from build123d import *

# Parameters (mm, degrees)
F0_W      = 116
F0_H      = 58
F1_DEPTH  = 80
F2_T      = -3
F4_DEPTH  = 47
F5_R      = 2
F6_DEPTH  = 3.001
F7_W      = 58
F7_H      = 4
F8_DEPTH  = 15
F9_R      = 10
F10_R     = 2
F11_DEPTH = 4.001
F12_W     = 48
F12_H     = 28.5
F13_DEPTH = 5
F14_R     = 1.875
F15_DEPTH = 5
F16_W     = 25
F16_H     = 5
F17_DEPTH = 5.001
F18_R     = 2.49999
F19_R     = 2.5
F20_SIZE  = 7


# Not quite as in the source:
# - a fillet or chamfer is up to 0.001 mm smaller than in the source, because OpenCascade refuses the exact size
# - a pattern or mirror of a feature is missing from the dataset's text; its kind, count and spacing are read off the source's solid


with BuildPart() as f1:
    # F0 (on Top) → F1 (new body)
    with BuildSketch(Plane.XY):
        Rectangle(F0_W, F0_H)
    extrude(amount=F1_DEPTH)

    # F2
    f2_openings = [f1.faces().sort_by_distance(p)[0] for p in [
        (0, 0, 80),
    ]]
    offset(amount=F2_T, openings=f2_openings)

    # F3 (on face) → F4 (join)
    with BuildSketch(Plane.XY.offset(3)):
        Polygon((-55, 26), (-55, 24), (53, 24), (53, -26), (55, -26), (55, 26), align=None)
    extrude(amount=F4_DEPTH)

    # F5 (on face) → F6 (cut, through all)
    with BuildSketch(Plane(origin=(55, 0, 0), x_dir=(0, -1, 0), z_dir=(-1, 0, 0))):
        with Locations((0, 69)):
            Circle(F5_R)
    extrude(amount=-F6_DEPTH, mode=Mode.SUBTRACT)

    # F7 (on face) → F8 (join)
    with BuildSketch(Plane.YZ.offset(58)):
        with Locations((0, 2)):
            Rectangle(F7_W, F7_H)
    f8 = extrude(amount=F8_DEPTH)

    # F8_copies: F8 across plane
    add(f8.mirror(Plane(origin=(0, 0, 0), x_dir=(0, 0, -1), z_dir=(-1, 0, 0))))

    # F9
    f9_edges = [f1.edges().sort_by_distance(p)[0] for p in [
        (73, 29, 2),
        (73, -29, 2),
        (-73, -29, 2),
        (-73, 29, 2),
    ]]
    fillet(f9_edges, radius=F9_R)

    # F10 (on face) → F11 (cut, through all)
    with BuildSketch(Plane.XY.offset(4)):
        with Locations((64.8827031255, 16)):
            Circle(F10_R)
        with Locations((64.8827031255, -16)):
            Circle(F10_R)
    f11 = extrude(amount=-F11_DEPTH, mode=Mode.SUBTRACT)

    # F11_copies: F11 across plane
    add(f11.mirror(Plane(origin=(0, 0, 0), x_dir=(0, 0, -1), z_dir=(-1, 0, 0))), mode=Mode.SUBTRACT)

    # F12 (on face) → F13 (cut)
    with BuildSketch(Plane.XZ.offset(29)):
        with Locations((-27, 26.25)):
            Rectangle(F12_W, F12_H)
    extrude(amount=-F13_DEPTH, mode=Mode.SUBTRACT)

    # F14 (on face) → F15 (cut)
    with BuildSketch(Plane.XZ.offset(29)):
        with Locations((-27, 47.1)):
            Circle(F14_R)
        with Locations((-27, 5.4)):
            Circle(F14_R)
    extrude(amount=-F15_DEPTH, mode=Mode.SUBTRACT)

    # F16 (on face) → F17 (cut, through all)
    with BuildSketch(Plane.XZ.offset(-24)):
        with Locations((20.5, 10.5)):
            Rectangle(F16_W, F16_H)
    extrude(amount=-F17_DEPTH, mode=Mode.SUBTRACT)

    # F18 (radius 2.5 in the source; OpenCascade refuses exactly that, so slightly less here)
    f18_edges = [f1.edges().sort_by_distance(p)[0] for p in [
        (33, 26.5, 13),
        (8, 26.5, 13),
        (33, 26.5, 8),
        (8, 26.5, 8),
    ]]
    fillet(f18_edges, radius=F18_R)

    # F19
    f19_edges = [f1.edges().sort_by_distance(p)[0] for p in [
        (-58, -29, 42),
        (58, -29, 42),
        (58, 29, 42),
        (-58, 29, 42),
    ]]
    fillet(f19_edges, radius=F19_R)

    # F20
    f20_edges = [f1.edges().sort_by_distance(p)[0] for p in [
        (-55, -1, 3),
        (53, -1, 3),
    ]]
    chamfer(f20_edges, length=F20_SIZE)


solid = f1.part
CAD build for the part. Positions are in the model's coordinates, mm. A direction names the side the tool comes from. Round coordinates to 2 decimals unless told otherwise and drop trailing zeros. Loops run counter-clockwise (first coordinate to the right, second up) from the corner with the lowest first, then second, coordinate; pieces in that order, holes last.
(1) Which spindle directions (+Z, -Z, +X, -X, +Y, -Y) get a long thin tool onto all of the face, cutting with end or side? Do faces 4 (the flat face through (20, 26, 13)), 5 (the cylindrical face through (56, 0, 71)), 6 (the flat face through (53, -1, 30)), 7 (the flat face through (-51, -28, 26)). Say none if no direction does.
(2) Cut at A-A (x = 26.5). Give the cut face in (y, z), plus the area to 3 significant figures.
(3) Cut at D-D (z = 23). Give the cut face in (x, y), plus the area to 3 significant figures.
(4) Cut at C-C (z = 73). Give the cut face in (x, y), plus the area to 3 significant figures.
(5) Two-plate mould, pull along Y, no slides. Class faces 1 (the flat face through (-1, 26, 65)), 2 (the cylindrical face through (-25.27, -27.52, 46.38)), 3 (the cylindrical face through (-69.99, -26.15, 2.03)): +Y half, -Y half, draft (parallel to the pull), parting line (faces both ways), or undercut.
(6) Cut at B-B (y = -16). Give the cut face in (x, z).
(7) Drop flat-ended pins along their axis: pin 1 (3.5 mm diameter, centred on x = -64.88, y = -16, fed in from -Z); pin 2 (4.5 mm diameter, centred on x = 64.88, y = 16, fed in from +Z); pin 3 (16 mm diameter, centred on y = 8, z = 47, fed in from -X); pin 4 (1.5 mm diameter, centred on y = -11.5, z = 68.5, fed in from +X). Give the stop position or say it passes through.
(8) Wall check: line 1 along X through (y, z) = (15, 47.5); line 2 along Y through (x, z) = (28, 38.5); line 3 along X through (y, z) = (-1.5, 59). Give the ranges that are in metal, low to high.
Findings below:
1. face 4: +Y
1. face 5: +X
1. face 6: +Z
1. face 7: -Y
2. outline: (-29, 0) - (29, 0) - (29, 8) - (24, 8) - (24, 3) - (-26, 3) - (-26, 80) - (-29, 80) - close; (24, 13) - (29, 13) - (29, 80) - (26, 80) - (26, 50) - (24, 50) - close
2. area: 705 mm2
3. outline: (-58, -26.5) arc R2.5 ccw to (-55.5, -29) - (-51, -29) - (-51, -26) - (-55, -26) - (-55, 24) - (53, 24) - (53, -26) - (-3, -26) - (-3, -29) - (55.5, -29) arc R2.5 ccw to (58, -26.5) - (58, 26.5) arc R2.5 ccw to (55.5, 29) - (-55.5, 29) arc R2.5 ccw to (-58, 26.5) - close
3. area: 1,180 mm2
4. outline: (-58, -26.5) arc R2.5 ccw to (-55.5, -29) - (55.5, -29) arc R2.5 ccw to (58, -26.5) - (58, 26.5) arc R2.5 ccw to (55.5, 29) - (-55.5, 29) arc R2.5 ccw to (-58, 26.5) - close; hole (-55, -26) - (55, -26) - (55, 26) - (-55, 26) - close
4. area: 1,000 mm2
5. face 1: undercut
5. face 2: draft
5. face 3: -Y half
6. outline: (-73, 0) - (-66.88, 0) - (-66.88, 4) - (-73, 4) - close; (-62.88, 0) - (62.88, 0) - (62.88, 4) - (58, 4) - (58, 80) - (55, 80) - (55, 50) - (53, 50) - (53, 10) - (46, 3) - (-48, 3) - (-55, 10) - (-55, 80) - (-58, 80) - (-58, 4) - (-62.88, 4) - close; (66.88, 0) - (73, 0) - (73, 4) - (66.88, 4) - close
7. pin 1: passes through
7. pin 2: stops at z = 4
7. pin 3: stops at x = -58
7. pin 4: stops at x = 58
8. line 1: x = -58 to -55, 53 to 58
8. line 2: y = -29 to -26, 24 to 29
8. line 3: x = -58 to -55, 55 to 58
